Design review of the part shown in the three views and the two pictorial views. Dimensions are in mm from the part's minimum x, y and z. Round coordinates to 2 decimals unless told otherwise and drop trailing zeros. Order: outer loops, then holes, each group sorted by start corner. A loop starts at its lowest first (then second) coordinate and runs counter-clockwise, first axis right, second up.
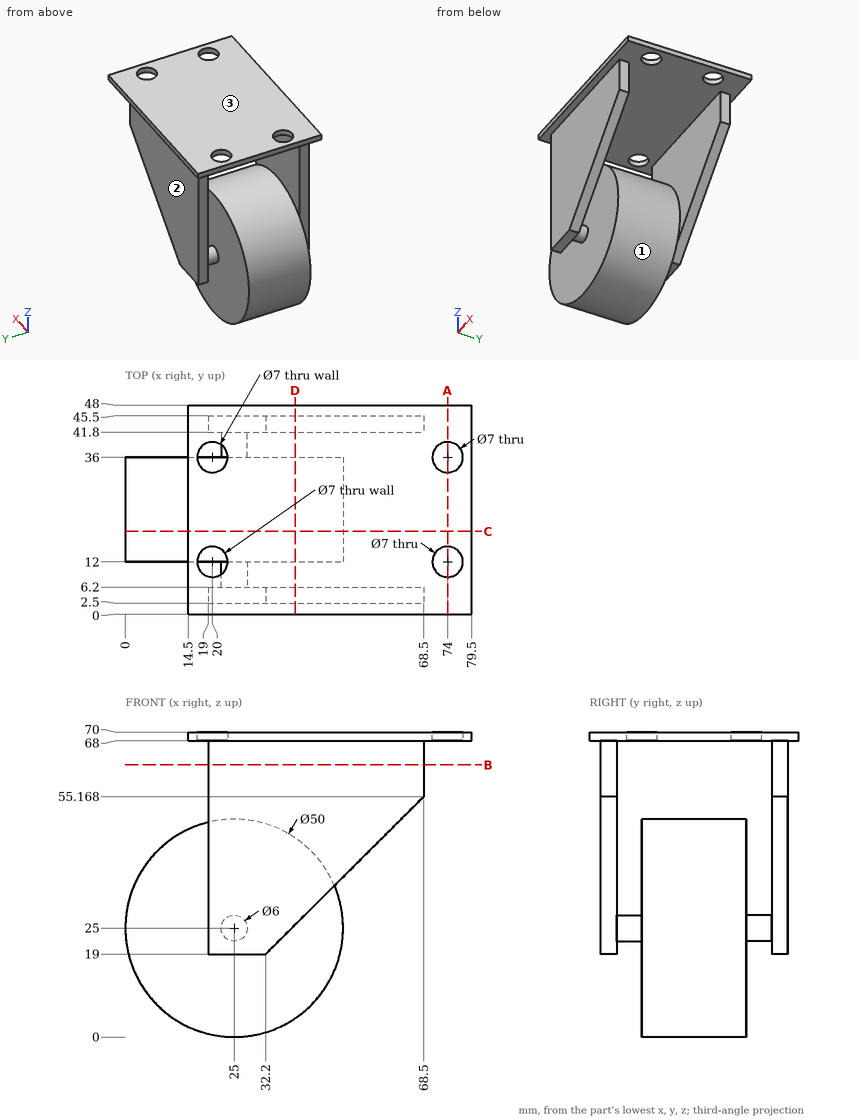
1) To check wall thickness, follow line 1 along Y through (x, z) = (20, 69.55); line 2 along Y through (x, z) = (62, 65.5); line 3 along Z through (x, y) = (68, 41.5). State the ranges of each line that lie inside material, in increasing order.
Results:
line 1: y = 0 to 8.5, 15.5 to 32.5, 39.5 to 48
line 2: y = 2.5 to 6.2, 41.8 to 45.5
line 3: z = 68 to 70
2) Take a section at D-D on x = 39. Give the boundary of the cut face in (y, z) (1 decimal), plus the area to 3 significant figures.
Results:
outline: (0, 68) - (2.5, 68) - (2.5, 25.8) - (6.2, 25.8) - (6.2, 68) - (41.8, 68) - (41.8, 25.8) - (45.5, 25.8) - (45.5, 68) - (48, 68) - (48, 70) - (0, 70) - close; (12, 4.3) - (36, 4.3) - (36, 45.7) - (12, 45.7) - close
area: 1,400 mm2
3) Take a section at A-A on x = 74. Give the boundary of the cut face in (y, z), plus the area to 3 significant figures.
Results:
outline: (0, 68) - (8.5, 68) - (8.5, 70) - (0, 70) - close; (15.5, 68) - (32.5, 68) - (32.5, 70) - (15.5, 70) - close; (39.5, 68) - (48, 68) - (48, 70) - (39.5, 70) - close
area: 68.0 mm2
4) Take a section at B-B on z = 62.5. Give the boundary of the cut face in (x, y), plus the area to 3 significant figures.
Results:
outline: (19, 2.5) - (68.5, 2.5) - (68.5, 6.2) - (19, 6.2) - close; (19, 41.8) - (68.5, 41.8) - (68.5, 45.5) - (19, 45.5) - close
area: 366 mm2
5) The part is to be moulded in two halves that separate along Z. For the marked faces 1, 2 and 3, say which applies: released by +Z, released by -Z, zero draft, split by the parting line, or undercut.
Results:
face 1: undercut
face 2: zero draft
face 3: released by +Z
6) Take a section at C-C on y = 19. Give the boundary of the cut face in (x, z), plus the area to 3 significant figures.
Results:
outline: circle Ø50 at (25, 25); (14.5, 68) - (79.5, 68) - (79.5, 70) - (14.5, 70) - close
area: 2,090 mm2
7) Clearance check with flat-ended pins moving along their axes: P1, Ø0.6, axis at y = 24.5, z = 69, coming from the -X side; P2, Ø5, axis at x = 43.5, z = 56.5, coming from the -Y side; P3, Ø4, axis at y = 3.5, z = 64.5, coming from the +X side. State where each tip first meets the part, or that it passes through.
Results:
P1: stops at x = 14.5
P2: stops at y = 2.5
P3: stops at x = 68.5
